Autodesk Inventor part; units mm, degrees
ref_plane "YZ Plane" through (0, 0, 0) normal (1, 0, 0) x (0, 1, 0)
ref_plane "XZ Plane" through (0, 0, 0) normal (0, 1, 0) x (-1, 0, 0)
ref_plane "XY Plane" through (0, 0, 0) normal (0, 0, 1) x (1, 0, 0)
sketch "草图1" plane through (0, 0, 0) normal (0, 0, 1) x (1, 0, 0)
  circle A0 centre (0, 0) radius 20
  circle A1 centre (0, 0) radius 35
  line L0 (-35, 0) -> (35, 0)
  point P0 (-20, 0)
  point P1 (20, 0)
  dimension "d0" = 70
  dimension "d1" = 70
extrude "拉伸1" add sketch "草图1" along normal mid plane 20 contours L0 A1 A0 picked at (-29.7075, -2.5961)
sketch "草图2" plane through (0, 0, 0) normal (0, 0, 1) x (1, 0, 0)
  line L0 (-20, 0) -> (-40, 0)
  line L1 (-40, 0) -> (-40, -30)
  line L2 (-40, -30) -> (-20, -30)
  line L3 (-20, -30) -> (-20, 0)
  line L4 (20, 0) -> (35, 0)
  line L5 (20, 0) -> (40, 0)
  line L6 (40, 0) -> (40, -30)
  line L7 (40, -30) -> (20, -30)
  line L8 (20, -30) -> (20, 0)
  point P0 (0, 0)
  dimension "d4" = 20
  dimension "d5" = 30
  dimension "d6" = 20
  dimension "d7" = 30
extrude "拉伸2" add sketch "草图2" along normal mid plane 30
sketch "草图3" plane through (-40, 0, -15) normal (0, 1, 0) x (1, 0, 0)
  line L0 (20, -5) -> (20, -25) construction
  line L1 (20, 0) -> (20, -5) construction
  line L2 (0, 0) -> (20, 0) construction
  line L3 (0, -30) -> (0, 0) construction
  line L4 (20, -30) -> (0, -30) construction
  line L5 (20, -25) -> (20, -30) construction
  point P0 (40, -15)
  point P1 (10, -15)
  point P2 (20, -15)
  point P3 (10, 0)
hole "孔1" at (-30, 0, 0) direction (0, -1, 0) diameter 10 end through all
mirror "镜像1" about plane through (0, 0, 0) normal (1, 0, 0) of "孔1"
properties part number "连接下环"
Source: CAD feature listing. Evaluate the final solid. Frame: model axes, mm. A direction names the side the tool comes from. Coordinates: 2 decimals unless noted, no trailing zeros. Loops run counter-clockwise (first coordinate to the right, second up) from the corner with the lowest first, then second, coordinate; pieces in that order, holes last. Notation, with made-up numbers: M 27.5,-6 L 32.5,-6 A24 cw 32.5,33 Z; hole C 17.5,81 d4. An arc over 180 degrees is marked long. Use CSV: the item, a comma, the result in double quotes.
(1) Draft query along Z for faces 1 (the face through (-30, -15, -15)), 2 (the face through (0, -25, 10)), 3 (the face through (-25.12, -15.21, -1.08)). Return one class per face: pulls with the +Z half, pulls with the -Z half, needs draft (parallel to the pull), parting line crosses it, or undercut.
Answers follow:
face 1,"pulls with the -Z half"
face 2,"pulls with the +Z half"
face 3,"undercut"
(2) Contact query for flat-ended pins moving along their axis: pin 1 (6 mm diameter, centred on x = 28, z = -3, fed in from -Y); pin 2 (17.5 mm diameter, centred on x = 6, y = -11, fed in from -Z); pin 3 (4 mm diameter, centred on x = 15.5, z = 2.5, fed in from +Y). Output: stop coordinate, or through.
Answers follow:
pin 1,"y = -30"
pin 2,"z = -10"
pin 3,"y = -9.68"
(3) Cut plane D-D on z = -12. Return loops of the section in (x, y).
Answers follow:
outline,"M -40,-30 L -20,-30 L -20,0 L -40,0 Z; M 20,-30 L 40,-30 L 40,0 L 20,0 Z"
(4) Cut plane C-C on x = -30. Return loops of the section in (y, z), and give its area (3 significant figures).
Answers follow:
outline,"M -30,-15 L 0,-15 L 0,-5 L -30,-5 Z; M -30,5 L 0,5 L 0,15 L -30,15 Z"
area,"600 mm²"
(5) Cut plane B-B on z = 0. Return loops of the section in (x, y).
Answers follow:
outline,"M -40,-30 L -35,-30 L -35,0 L -40,0 Z; M -25,-30 L -20,-30 L -20,-28.72 A35 ccw 20,-28.72 L 20,-30 L 25,-30 L 25,0 L 20,0 A20 cw -20,0 L -25,0 Z; M 35,-30 L 40,-30 L 40,0 L 35,0 Z"
(6) Line query: line 1 (X direction, y = -23.5, z = 0); line 2 (Z direction, x = 30, y = -7); line 3 (X direction, y = -5, z = -11.5). Output: solid intervals per line, ascending. Write a range as [from, to].
Answers follow:
line 1,"[-40, -35], [-25, 25], [35, 40]"
line 2,"[-15, -5], [5, 15]"
line 3,"[-40, -20], [20, 40]"
(7) Reachability of faces 4 (the face through (0, -25, -10)), 5 (the face through (30, -15, 15)), 6 (the face through (-35, -30, -4)), 7 (the face through (35, -30, -4)) from +Z, -Z, +X, -X, +Y, -Y: full face, straight path, thin tool, end or side. Return the list, or none.
Answers follow:
face 4,"-Z, +Y, -Y"
face 5,"+Z, +X, -X, +Y, -Y"
face 6,"+Z, -Z, -X, -Y"
face 7,"+Z, -Z, +X, -Y"
(8) Cut plane A-A on y = -16. Return loops of the section in (x, z), and give its area (3 significant figures).
Answers follow:
outline,"M -40,-15 L -20,-15 L -20,-10 L -12,-10 L -12,10 L -20,10 L -20,15 L -40,15 Z; M 12,-10 L 20,-10 L 20,-15 L 40,-15 L 40,15 L 20,15 L 20,10 L 12,10 Z; hole C -30,0 d10; hole C 30,0 d10"
area,"1,360 mm²"
